```python
from build123d import *

# Parameters (mm, degrees)
BOSS_EXTRUDE1_DEPTH = 5


with BuildPart() as part:
    # Sketch1 → Boss-Extrude1 (new body)
    with BuildSketch(Plane(origin=(0, 0, 0), x_dir=(1, 0, 0), z_dir=(0, 1, 0))):
        with BuildLine():
            Line((-135, 2), (-135, -2))
            Line((-135, -2), (-130.968871126, -2))
            ThreePointArc((-130.968871126, -2), (-130.61878556, -1.027112473), (-130.5, 0))
            ThreePointArc((-130.5, 0), (-130.61878556, 1.027112473), (-130.968871126, 2))
            Line((-130.968871126, 2), (-135, 2))
        make_face()
        with BuildLine():
            Line((-130.968871126, -2), (-135, -2))
            Line((-135, -2), (-135, 2))
            Line((-135, 2), (-130.968871126, 2))
            ThreePointArc((-130.968871126, 2), (-139.5, 0), (-130.968871126, -2))
        make_face()
        with BuildLine():
            ThreePointArc((-130.5, 0), (-130.61878556, -1.027112473), (-130.968871126, -2))
            Line((-130.968871126, -2), (130.968871126, -2))
            ThreePointArc((130.968871126, -2), (130.5, 0), (130.968871126, 2))
            Line((130.968871126, 2), (-130.968871126, 2))
            ThreePointArc((-130.968871126, 2), (-130.61878556, 1.027112473), (-130.5, 0))
        make_face()
        with BuildLine():
            ThreePointArc((130.968871126, 2), (130.5, 0), (130.968871126, -2))
            Line((130.968871126, -2), (135, -2))
            Line((135, -2), (135, 2))
            Line((135, 2), (130.968871126, 2))
        make_face()
        with BuildLine():
            Line((135, -2), (130.968871126, -2))
            ThreePointArc((130.968871126, -2), (136.027112473, -4.38121444), (139.5, 0))
            ThreePointArc((139.5, 0), (136.027112473, 4.38121444), (130.968871126, 2))
            Line((130.968871126, 2), (135, 2))
            Line((135, 2), (135, -2))
        make_face()
    extrude(amount=BOSS_EXTRUDE1_DEPTH)

    # Cut-Sweep1: sweep along a path in Sketch2
    with BuildLine(Plane(origin=(0, 5, 0), x_dir=(1, 0, 0), z_dir=(0, 1, 0))) as cut_sweep1_path:
        CenterArc((-135, 0), 4.5, 0, 360)
    # 3DSketch1 → Cut-Sweep1 (sweep, cut)
    with BuildSketch(Plane(origin=(-135, 5, 0), x_dir=(0, -1, 0), z_dir=(-1, 0, 0))):
        with BuildLine():
            Line((0, 0), (-1.5, 0))
            ThreePointArc((-1.5, 0), (1.25, -2.75), (4, 0))
            Line((4, 0), (0, 0))
        make_face()
    cut_sweep1 = sweep(path=cut_sweep1_path.line, mode=Mode.SUBTRACT)

    # Mirror1: Cut-Sweep1 across plane
    add(cut_sweep1.mirror(Plane(origin=(0, 0, 0), x_dir=(0, 0, 1), z_dir=(1, 0, 0))), mode=Mode.SUBTRACT)


solid = part.part
```
For this review, take the finished solid that the model builds, in its own axes (mm). A direction names the side the tool comes from. Round coordinates to 2 decimals unless told otherwise and drop trailing zeros. Write each loop counter-clockwise with the first axis right and the second up, starting at its lowest first coordinate (ties: lowest second). Pieces come first, ordered by that corner, then holes. Notation, with made-up numbers: (19.25, 38) -> (39.25, 38) arc R17 ccw to (39.25, 65) -> close; hole circle Ø5 at (-21, 76). An arc over 180 degrees is marked (long way). One line per question, with ' | ' between items. Start each with the question number.
(1) Tool access review of faces 1 (the face through (-2, 2, 2)), 2 (the face through (2, 2, -2)), 3 (the face through (-2, 5, 1)): name each direction out of +Z, -Z, +X, -X, +Y, -Y from which nothing blocks a thin tool from reaching the whole face with its end or side.
(2) For line 1 along X through (y, z) = (2.25, 0); line 2 along Z through (x, y) = (-94, 0.55); line 3 along X through (y, z) = (3.5, 0.5), list the stretches that pass through material, from the lowest coordinate up. Write a range as from..to.
(3) Add section B-B, the plane x = -104. Write out the cut boundary in (y, z), plus the area to 3 significant figures.
(4) Add section A-A, the plane y = 2.45. Write out the cut boundary in (x, z).
(5) Insertion check: P1, Ø1.5, axis at x = -0.5, y = 2, coming from the +Z side; P2, Ø2, axis at y = 2, z = -3, coming from the -X side; P3, Ø1.5, axis at x = -51.5, y = 2.5, coming from the -Z side. Each pin has a flat end and moves straight along its axis. Give the tip position at first contact, or say it passes through.
(6) Add section C-C, the plane x = -135. Write out the cut boundary in (y, z), plus the area to 3 significant figures.
(7) Mouldability with a two-part tool opening along X and no side actions: class faces 4 (the face through (-2, 0, 1)), 5 (the face through (-139.497, 2.465, -0.169)) as released by +X, released by -X, zero draft, split by the parting line, or undercut.
Answer list:
1) face 1: +Z, +Y, -Y | face 2: -Z, +Y, -Y | face 3: +Z, -Z, +X, -X, +Y
2) line 1: -139.5..-137.3, -132.7..132.7, 137.3..139.5 | line 2: -2..2 | line 3: -139.47..-137.69, -132.31..132.31, 137.69..139.47
3) outline: (0, -2) -> (5, -2) -> (5, 2) -> (0, 2) -> close | area: 20.0 mm²
4) outline: (-130.97, -2) -> (130.97, -2) arc R4.5 ccw (long way) to (130.97, 2) -> (-130.97, 2) arc R4.5 ccw (long way) to start; hole circle Ø4.85 at (-135, 0); hole circle Ø4.85 at (135, 0)
5) P1: z = 2 | P2: x = -139.03 | P3: z = -2
6) outline: (0, -4.5) -> (5, -4.5) -> (5, -2.45) arc R2.75 cw (long way) to (5, 2.45) -> (5, 4.5) -> (0, 4.5) -> close | area: 26.5 mm²
7) face 4: zero draft | face 5: undercut
